from build123d import *

# Parameters (mm, degrees)
F0_R     = 10.16
F1_DEPTH = 15.7734
F2_R     = 28.575
F3_DEPTH = 40.2336
F5_DEPTH = 40.2346
F6_R     = 3.302


with BuildPart() as f1:
    # F0 (on Top) → F1 (new body)
    with BuildSketch(Plane.XY):
        with BuildLine():
            Line((9.559057, 26.928703), (0, 28.575))
            ThreePointArc((0, 28.575), (-28.575, 0), (0, -28.575))
            Line((0, -28.575), (9.559057, -26.928703))
            ThreePointArc((9.559057, -26.928703), (23.341815, -16.48303), (28.575, 0))
            ThreePointArc((28.575, 0), (23.341815, 16.48303), (9.559057, 26.928703))
        make_face()
        with BuildLine():
            ThreePointArc((13.447765, -4.826), (-14.2875, 0), (13.447765, 4.826))
            Line((13.447765, 4.826), (18.5293, 4.826))
            Line((18.5293, 4.826), (18.5293, 0))
            Line((18.5293, 0), (18.5293, -4.826))
            Line((18.5293, -4.826), (13.447765, -4.826))
        make_face(mode=Mode.SUBTRACT)
        with BuildLine():
            ThreePointArc((9.559057, 26.928703), (4.849894, 28.160418), (0, 28.575))
            Line((0, 28.575), (9.559057, 26.928703))
        make_face()
        with BuildLine():
            Line((9.559057, -26.928703), (0, -28.575))
            ThreePointArc((0, -28.575), (4.849894, -28.160418), (9.559057, -26.928703))
        make_face()
        with BuildLine():
            Line((55.833732, 18.959104), (9.559057, 26.928703))
            ThreePointArc((9.559057, 26.928703), (23.341815, 16.48303), (28.575, 0))
            ThreePointArc((28.575, 0), (23.341815, -16.48303), (9.559057, -26.928703))
            Line((9.559057, -26.928703), (55.833732, -18.959104))
            ThreePointArc((55.833732, -18.959104), (73.025, 0), (55.833732, 18.959104))
        make_face()
        with Locations((53.975, 0)):
            Circle(F0_R, mode=Mode.SUBTRACT)
    extrude(amount=F1_DEPTH)

    # F2 (on Top) → F3 (join)
    with BuildSketch(Plane.XY):
        Circle(F2_R)
    extrude(amount=F3_DEPTH)

    # F4 (on Top) → F5 (cut, through all)
    with BuildSketch(Plane.XY):
        with BuildLine():
            Line((18.5293, 4.826), (13.447765, 4.826))
            ThreePointArc((13.447765, 4.826), (-14.2875, 0), (13.447765, -4.826))
            Line((13.447765, -4.826), (18.5293, -4.826))
            Line((18.5293, -4.826), (18.5293, 0))
            Line((18.5293, 0), (18.5293, 4.826))
        make_face()
    extrude(amount=F5_DEPTH, mode=Mode.SUBTRACT)

    # F6
    f6_edges = [f1.edges().sort_by_distance(p)[0] for p in [
        (-28.575, 0, 40.2336),
    ]]
    fillet(f6_edges, radius=F6_R)


solid = f1.part
Geometry check sheet. Reference: the model listing, model coordinates, mm. A direction names the side the tool comes from. Give positions to 0.01 mm unless a question says otherwise; leave off trailing zeros. Order: outer loops, then holes, each group sorted by start corner. A loop starts at its lowest first (then second) coordinate and runs counter-clockwise, first axis right, second up. Notation, with made-up numbers: M -5,-14.5 L 26,-14.5 A33 cw 26,15.5 Z; hole C -23.75,-32 d10. An arc over 180 degrees is marked long. Use a Markdown table: item, result.
Item 1: Section check A-A (y = 0). Record the cut outline in (x, z) (1 decimal).
Answers follow:
| item | result |
|---|---|
| outline | M -28.6,0 L -14.3,0 L -14.3,40.2 L -25.3,40.2 A3.3 ccw -28.6,36.9 Z; M 18.5,0 L 43.8,0 L 43.8,15.8 L 28.6,15.8 L 28.6,36.9 A3.3 ccw 25.3,40.2 L 18.5,40.2 Z; M 64.1,0 L 73,0 L 73,15.8 L 64.1,15.8 Z |
Item 2: Draft check along X on faces 1 (the flat face through (41, 0, 15.773)), 2 (the cylindrical face through (73.02, -0.39, 7.78)), 3 (the flat face through (18.529, 0, 20)), 4 (the flat face through (16, 4.826, 20)). Enter one of: +X half, -X half, draft (parallel to the pull), parting line (faces both ways), or undercut.
Answers follow:
| item | result |
|---|---|
| face 1 | draft |
| face 2 | +X half |
| face 3 | undercut |
| face 4 | undercut |
Item 3: Depth check by flat-ended pin: P1, Ø4, axis at y = 21.5, z = 32.5, coming from the -X side; P2, Ø5.5, axis at x = 17, z = 20.5, coming from the -Y side; P3, Ø1.5, axis at y = 18, z = 14.5, coming from the +X side; P4, Ø10, axis at x = 38, z = 29, coming from the +Y side. Enter the tip coordinate at first touch or a pass-through.
Answers follow:
| item | result |
|---|---|
| P1 | stops at x = -20.89 |
| P2 | stops at y = -24.77 |
| P3 | stops at x = 62.06 |
| P4 | passes through |
Item 4: Material ranges on line 1 along X through (y, z) = (0, 32.5) (1 decimal); line 2 along X through (y, z) = (-2.5, 14); line 3 along Z through (x, y) = (63.5, -11), recorded low to high.
Answers follow:
| item | result |
|---|---|
| line 1 | x = -28.6 to -14.3, 18.5 to 28.6 |
| line 2 | x = -28.47 to -14.07, 18.53 to 44.13, 63.82 to 72.86 |
| line 3 | z = 0 to 15.77 |
Item 5: Section check C-C (x = 33). Record the cut outline in (y, z), and give its area (3 significant figures).
Answers follow:
| item | result |
|---|---|
| outline | M -22.89,0 L 22.89,0 L 22.89,15.77 L -22.89,15.77 Z |
| area | 722 mm2 |
Item 6: Tool access check on faces 5 (the flat face through (22, 0, 0)), 6 (the flat face through (16, -4.826, 20)). Record the directions out of +Z, -Z, +X, -X, +Y, -Y that give a thin tool (end or side, any length) a straight path to the whole face; none if there is none.
Answers follow:
| item | result |
|---|---|
| face 5 | -Z, +X, -X, +Y, -Y |
| face 6 | +Z, -Z |
